```python
from build123d import *

# Parameters (mm, degrees)
BOSS_EXTRUDE1_START = -6.63575
SKETCH4_R           = 10.7188
BOSS_EXTRUDE1_DEPTH = 6.63575
SKETCH5_W           = 6.63575
SKETCH5_H           = 0.254
CUT_EXTRUDE1_START  = 26.19375
SKETCH6_R           = 1.984375
CUT_EXTRUDE1_DEPTH  = 50.8


with BuildPart() as part:
    # Sketch3 → Revolve1 (revolve)
    with BuildSketch(Plane(origin=(0, 0, 0), x_dir=(0, 0, -1), z_dir=(1, 0, 0)), mode=Mode.PRIVATE) as revolve1_sk:
        with BuildLine():
            Line((6.461125, 0), (13.096875, 0))
            Line((13.096875, 0), (13.096875, -10.7188))
            Line((13.096875, -10.7188), (-13.096875, -10.7188))
            Line((-13.096875, -10.7188), (-13.096875, -7.9502))
            Line((-13.096875, -7.9502), (4.873625, -7.9502))
            ThreePointArc((4.873625, -7.9502), (6.060370876, -4.053573618), (6.461125, 0))
        make_face()
    revolve(revolve1_sk.sketch.rotate(Axis((0, 0, 13.096875), (0, 0, -1)), 270), axis=Axis((0, 0, 13.096875), (0, 0, -1)))

    # Sketch4 → Boss-Extrude1 (add)
    with BuildSketch(Plane(origin=(0, 0, -13.096875), x_dir=(-1, 0, 0), z_dir=(0, 0, -1)).offset(BOSS_EXTRUDE1_START)):
        Polygon((4.99748663, 12.065), (-4.99748663, 12.065), (-12.065, 4.99748663), (-12.065, -4.99748663), (-4.99748663, -12.065), (4.99748663, -12.065), (12.065, -4.99748663), (12.065, 4.99748663), align=None)
        with Locations(Location((0, 0, 0), (0, 0, 180))):
            Circle(SKETCH4_R, mode=Mode.SUBTRACT)
    extrude(amount=BOSS_EXTRUDE1_DEPTH)

    # Sketch5 → Cut-Revolve1 (revolve, cut)
    with BuildSketch(Plane(origin=(0, 0, 0), x_dir=(0, 0, -1), z_dir=(0.9238795325112871, -0.3826834323650893, 0)), mode=Mode.PRIVATE) as cut_revolve1_sk:
        with Locations((9.779, 12.932061897)):
            Rectangle(SKETCH5_W, SKETCH5_H)
    revolve(cut_revolve1_sk.sketch.rotate(Axis((0, 0, 13.096875), (0, 0, 1)), 202.5), axis=Axis((0, 0, 13.096875), (0, 0, 1)), mode=Mode.SUBTRACT)

    # Sketch6 → Cut-Extrude1 (cut)
    with BuildSketch(Plane(origin=(-8.103148128, -57.606298873, -13.096875), x_dir=(1, 0, 0), z_dir=(0, 0, 1)).offset(CUT_EXTRUDE1_START)):
        with Locations(Location((8.103148128, 57.606298873, 0), (0, 0, 270))):
            Circle(SKETCH6_R)
    extrude(amount=-CUT_EXTRUDE1_DEPTH, mode=Mode.SUBTRACT)


solid = part.part
```
Geometry check sheet. Reference: the model listing, model coordinates, mm. A direction names the side the tool comes from. Give positions to 0.01 mm unless a question says otherwise; leave off trailing zeros. Loops run counter-clockwise (first coordinate to the right, second up) from the corner with the lowest first, then second, coordinate; pieces in that order, holes last. Notation, with made-up numbers: M 59.25,48.25 L 105.25,48.25 A15 cw 105.25,63.25 Z; hole C 80,63.25 d7. An arc over 180 degrees is marked long. Write item = value, one per line. Start each with the question number.
1. Section check A-A, the plane x = 0. Enter the section's corners in (y, z) (3 decimals), plus the area to 3 significant figures.
2. Thickness scan on probe 1 along Y at (x, z) = (0, 0.75); probe 2 along Y at (x, z) = (0, -9.25) (3 decimals); probe 3 along Z at (x, y) = (-0.5, -10.75). Record the ranges inside material, lowest first.
3. Tool access check on faces 4 (the face through (-4.892, 11.834, -9.825)), 5 (the face through (-1.395, -10.628, 3.455)). Record the directions out of +Z, -Z, +X, -X, +Y, -Y that give a thin tool (end or side, any length) a straight path to the whole face; none if there is none.
4. Draft check along Y on faces 1 (the face through (-4.909, -11.827, -9.825)), 2 (the face through (4.909, 11.827, -9.825)), 3 (the face through (-1.937, 0.43, -9.684)). Enter one of: +Y half, -Y half, draft (parallel to the pull), parting line (faces both ways), or undercut.
5. Go/stop test with flat-tipped pins: P1, Ø12.5, axis at x = 0, y = 0, coming from the -Z side; P2, Ø8, axis at y = -7, z = 9.5, coming from the -X side; P3, Ø6, axis at x = 3.5, z = 9.5, coming from the +Y side; P4, Ø3, axis at y = -5, z = 7, coming from the -X side. Record where each tip stops, or that it passes through.
6. Section check D-D, the plane y = 7. Enter the section's corners in (x, z), plus the area to 3 significant figures.
7. Section check B-B, the plane z = -9.25. Enter the section's corners in (x, y) (3 decimals), plus the area to 3 significant figures.
Values follow:
q1.outline = M -12.065,-13.097 L -1.984,-13.097 L -1.984,-6.366 A20.701 cw -7.95,-4.874 L -7.95,13.097 L -10.719,13.097 L -10.719,-6.461 L -12.065,-6.461 Z; M 1.984,-13.097 L 12.065,-13.097 L 12.065,-6.461 L 10.719,-6.461 L 10.719,13.097 L 7.95,13.097 L 7.95,-4.874 A20.701 cw 1.984,-6.366 Z
q1.area = 250 mm^2
q2.probe_1 = -10.72 to -7.95, 7.95 to 10.72
q2.probe_2 = -12.065 to -1.984, 1.984 to 12.065
q2.probe_3 = -13.1 to -6.46
q3.face_4 = +Z, -Z, -X, +Y
q3.face_5 = +Z
q4.face_1 = -Y half
q4.face_2 = +Y half
q4.face_3 = undercut
q5.P1 = -13.1
q5.P2 = -10.29
q5.P3 = 10.71
q5.P4 = -10.13
q6.outline = M -10.06,-13.1 L 10.06,-13.1 L 10.06,-6.46 L 8.12,-6.46 L 8.12,13.1 L 3.77,13.1 L 3.77,-4.87 A19.48 cw -3.77,-4.87 L -3.77,13.1 L -8.12,13.1 L -8.12,-6.46 L -10.06,-6.46 Z
q6.area = 314 mm^2
q7.outline = M -12.065,-4.29 A12.805 ccw -11.565,-5.498 L -5.498,-11.565 A12.805 ccw -4.29,-12.065 L 4.29,-12.065 A12.805 ccw 5.498,-11.565 L 11.565,-5.498 A12.805 ccw 12.065,-4.29 L 12.065,4.29 A12.805 ccw 11.565,5.498 L 5.498,11.565 A12.805 ccw 4.29,12.065 L -4.29,12.065 A12.805 ccw -5.498,11.565 L -11.565,5.498 A12.805 ccw -12.065,4.29 Z; hole C 0,0 d3.969
q7.area = 469 mm^2
